For this review, take the finished solid that the model builds, in its own axes (mm). A direction names the side the tool comes from. Round coordinates to 2 decimals unless told otherwise and drop trailing zeros. Order: outer loops, then holes, each group sorted by start corner. A loop starts at its lowest first (then second) coordinate and runs counter-clockwise, first axis right, second up. Notation, with made-up numbers: (-18, -25) -> (23, -25) arc R37 ccw to (23, 11) -> close; hole circle Ø8 at (-30.5, -33.5). An arc over 180 degrees is marked (long way). Put each result on its own line as item: value. Start each with the question number.
Autodesk Inventor part; units mm, degrees
ref_plane "YZ Plane" through (0, 0, 0) normal (1, 0, 0) x (0, 1, 0)
ref_plane "XZ Plane" through (0, 0, 0) normal (0, 1, 0) x (-1, 0, 0)
ref_plane "XY Plane" through (0, 0, 0) normal (0, 0, 1) x (1, 0, 0)
sketch "Náčrt1" plane through (0, 0, 0) normal (0, 1, 0) x (-1, 0, 0)
  line L0 (0, 0) -> (0, 12)
  line L1 (0, 12) -> (1, 12)
  arc A0 (2.79, 0) -> (1, 12) centre (-37.5014, 0.1235) ccw
  line L2 (2.79, 0) -> (0, 0)
  dimension "d0" = 12
  dimension "d1" = 1
revolve "Rotace1" add sketch "Náčrt1" angle 360 about axis through (-2.79, 0, 0) along (1, 0, 0)
sketch "Náčrt2" plane through (0, 0, 0) normal (1, 0, 0) x (0, 0, -1)
  line L0 (-5.29, 5.29) -> (5.29, 5.29)
  line L1 (5.29, 5.29) -> (5.29, -5.29)
  line L2 (5.29, -5.29) -> (-5.29, -5.29)
  line L3 (-5.29, -5.29) -> (-5.29, 5.29)
  point P0 (0, 0)
  dimension "d3" = 10.58
  dimension "d4" = 10.58
  dimension "d5" = 5.29
  dimension "d6" = 5.29
extrude "Vysunutí1" add sketch "Náčrt2" along normal blind 6.6
sketch "Náčrt3" plane through (6.6, 0, 0) normal (1, 0, 0) x (0, 0, -1)
  circle A0 centre (0, 0) radius 5
  dimension "d9" = 10
extrude "Vysunutí2" add sketch "Náčrt3" along normal blind 63.4
chamfer "Zkosení1" distance 1 angle 45 1 edges at (70, 0, 5)
fillet "Zaoblení1" radius 1 4 edges at (6.6, 5.29, 0) (6.6, 0, 5.29) (6.6, -5.29, 0) (6.6, 0, -5.29)
thread "Závit1"
properties part number "Šroub M10x70"
Item 1: Consider section A-A, the plane x = 14. Write out the cut boundary in (y, z).
Item 2: For L1, parallel to Z at x = 2.5, y = -0.25; L2, parallel to Z at x = 53, y = -4, list the stretches that pass through material, from the lowest coordinate up.
Item 3: Insertion check: pin 1 Ø10 at (x, z) = (30, 4) entering from -Y; pin 2 Ø5 at (x, z) = (25, -4.5) entering from -Y; pin 3 Ø1.4 at (y, z) = (-3.5, 3.5) entering from +X; pin 4 Ø1.9 at (y, z) = (3.5, 3) entering from +X. Each pin has a flat end and moves straight along its axis. Give the tip position at first contact, or say it passes through.
Item 4: Tool access review of faces 1 (the face through (3, -5.29, 0)), 2 (the face through (6.6, -4, -4)), 3 (the face through (6.6, 4, -4)), 4 (the face through (6.6, 4, 4)), 5 (the face through (0, 0, -6)): name each direction out of +Z, -Z, +X, -X, +Y, -Y from which nothing blocks a thin tool from reaching the whole face with its end or side.
Evaluation:
1. outline: circle Ø10 at (0, 0)
2. L1: z = -5.29 to 5.29
2. L2: z = -3 to 3
3. pin 1: stops at y = -5
3. pin 2: stops at y = -4.58
3. pin 3: stops at x = 69.75
3. pin 4: stops at x = 70
4. face 1: +Z, -Z, +X, -Y
4. face 2: -Z, +X, -Y
4. face 3: -Z, +X, +Y
4. face 4: +Z, +X, +Y
4. face 5: +X
